```python
from build123d import *

# Parameters (mm, degrees)
F1_DEPTH = 15.875


with BuildPart() as f1:
    # F0 (on Front) → F1 (new body, symmetric)
    with BuildSketch(Plane.XZ):
        with BuildLine():
            Line((-43.1179597079, -20.6795539033), (-35.6798299226, -32.0231574202))
            ThreePointArc((-35.6798299226, -32.0231574202), (-28.999387078, -31.3506516016), (-25.4497350562, -37.0498226993))
            ThreePointArc((-25.4497350562, -37.0498226993), (-25.6219242672, -38.5185479478), (-26.1291535934, -39.9076200809))
            Line((-26.1291535934, -39.9076200809), (-15.6603085893, -45.1835936364))
            ThreePointArc((-15.6603085893, -45.1835936364), (-8.6969613087, -41.8243775437), (-3.6499608348, -47.681025418))
            Line((-3.6499608348, -47.681025418), (9.0295717487, -46.960294218))
            ThreePointArc((9.0295717487, -46.960294218), (13.3803993428, -40.5694541047), (20.6795539033, -43.1179597079))
            Line((20.6795539033, -43.1179597079), (31.2999856287, -36.1540218876))
            ThreePointArc((31.2999856287, -36.1540218876), (31.872492796, -28.4439782009), (39.4679988731, -27.0014715148))
            Line((39.4679988731, -27.0014715148), (45.1835936364, -15.6603085893))
            ThreePointArc((45.1835936364, -15.6603085893), (41.8243775437, -8.6969613087), (47.681025418, -3.6499608348))
            Line((47.681025418, -3.6499608348), (46.960294218, 9.0295717487))
            ThreePointArc((46.960294218, 9.0295717487), (40.5694541047, 13.3803993428), (43.1179597079, 20.6795539033))
            Line((43.1179597079, 20.6795539033), (36.1540218876, 31.2999856287))
            ThreePointArc((36.1540218876, 31.2999856287), (28.4439782009, 31.872492796), (27.0014715148, 39.4679988731))
            Line((27.0014715148, 39.4679988731), (15.6603085893, 45.1835936364))
            ThreePointArc((15.6603085893, 45.1835936364), (8.6969613087, 41.8243775437), (3.6499608348, 47.681025418))
            Line((3.6499608348, 47.681025418), (-9.0295717487, 46.960294218))
            ThreePointArc((-9.0295717487, 46.960294218), (-9.0218969832, 46.7801840579), (-9.0193380405, 46.599928618))
            ThreePointArc((-9.0193380405, 46.599928618), (-13.5523860225, 40.5154249107), (-20.6795539033, 43.1179597079))
            Line((-20.6795539033, 43.1179597079), (-31.2999856287, 36.1540218876))
            ThreePointArc((-31.2999856287, 36.1540218876), (-30.5256977842, 34.4890049955), (-30.2602014915, 32.6720529775))
            ThreePointArc((-30.2602014915, 32.6720529775), (-33.2803751727, 27.2651354928), (-39.4679988731, 27.0014715148))
            Line((-39.4679988731, 27.0014715148), (-45.1835936364, 15.6603085893))
            ThreePointArc((-45.1835936364, 15.6603085893), (-42.6344735333, 13.3195534454), (-41.691391018, 9.9897271266))
            ThreePointArc((-41.691391018, 9.9897271266), (-43.4256125593, 5.6288683556), (-47.681025418, 3.6499608348))
            Line((-47.681025418, 3.6499608348), (-46.960294218, -9.0295717487))
            ThreePointArc((-46.960294218, -9.0295717487), (-42.2390698471, -10.7535595818), (-40.249928618, -15.3693380405))
            ThreePointArc((-40.249928618, -15.3693380405), (-41.0127556934, -18.3869527791), (-43.1179597079, -20.6795539033))
        make_face()
        with BuildLine():
            ThreePointArc((-40.5228638212, 27.6706958124), (-43.8188886794, 22.0833623778), (-46.3490638812, 16.1100644426))
            ThreePointArc((-46.3490638812, 16.1100644426), (-45.7552417742, 15.9139166606), (-45.1835936364, 15.6603085893))
            Line((-45.1835936364, 15.6603085893), (-39.4679988731, 27.0014715148))
            ThreePointArc((-39.4679988731, 27.0014715148), (-40.0119284743, 27.3100800632), (-40.5228638212, 27.6706958124))
        make_face()
        with BuildLine():
            ThreePointArc((-21.2584815971, 44.2249574245), (-26.9065895731, 41.0341971599), (-32.0844345415, 37.1262570045))
            ThreePointArc((-32.0844345415, 37.1262570045), (-31.6682434024, 36.6594769889), (-31.2999856287, 36.1540218876))
            Line((-31.2999856287, 36.1540218876), (-20.6795539033, 43.1179597079))
            ThreePointArc((-20.6795539033, 43.1179597079), (-20.9963064816, 43.6571873513), (-21.2584815971, 44.2249574245))
        make_face()
        with BuildLine():
            ThreePointArc((3.7020936033, 48.9291774094), (-2.7846915195, 48.9899519509), (-9.2228068767, 48.1944989841))
            ThreePointArc((-9.2228068767, 48.1944989841), (-9.0957647853, 47.582160063), (-9.0295717487, 46.960294218))
            Line((-9.0295717487, 46.960294218), (3.6499608348, 47.681025418))
            ThreePointArc((3.6499608348, 47.681025418), (3.6452588769, 48.3063865448), (3.7020936033, 48.9291774094))
        make_face()
        with BuildLine():
            ThreePointArc((16.1100644426, 46.3490638812), (15.9139166606, 45.7552417742), (15.6603085893, 45.1835936364))
            Line((15.6603085893, 45.1835936364), (27.0014715148, 39.4679988731))
            ThreePointArc((27.0014715148, 39.4679988731), (27.3100800632, 40.0119284743), (27.6706958124, 40.5228638212))
            ThreePointArc((27.6706958124, 40.5228638212), (22.0833623778, 43.8188886794), (16.1100644426, 46.3490638812))
        make_face()
        with BuildLine():
            Line((36.1540218876, 31.2999856287), (43.1179597079, 20.6795539033))
            ThreePointArc((43.1179597079, 20.6795539033), (43.6571873513, 20.9963064816), (44.2249574245, 21.2584815971))
            ThreePointArc((44.2249574245, 21.2584815971), (41.0341971599, 26.9065895731), (37.1262570045, 32.0844345415))
            ThreePointArc((37.1262570045, 32.0844345415), (36.6594769889, 31.6682434024), (36.1540218876, 31.2999856287))
        make_face()
        with BuildLine():
            Line((46.960294218, 9.0295717487), (47.681025418, -3.6499608348))
            ThreePointArc((47.681025418, -3.6499608348), (48.3063865448, -3.6452588769), (48.9291774094, -3.7020936033))
            ThreePointArc((48.9291774094, -3.7020936033), (49.0340558686, -1.8523671577), (49.0690319755, 0))
            ThreePointArc((49.0690319755, 0), (48.8499094713, 4.6320884771), (48.1944989841, 9.2228068767))
            ThreePointArc((48.1944989841, 9.2228068767), (47.582160063, 9.0957647853), (46.960294218, 9.0295717487))
        make_face()
        with BuildLine():
            Line((45.1835936364, -15.6603085893), (39.4679988731, -27.0014715148))
            ThreePointArc((39.4679988731, -27.0014715148), (40.0119284743, -27.3100800632), (40.5228638212, -27.6706958124))
            ThreePointArc((40.5228638212, -27.6706958124), (43.8188886794, -22.0833623778), (46.3490638812, -16.1100644426))
            ThreePointArc((46.3490638812, -16.1100644426), (45.7552417742, -15.9139166606), (45.1835936364, -15.6603085893))
        make_face()
        with BuildLine():
            Line((31.2999856287, -36.1540218876), (20.6795539033, -43.1179597079))
            ThreePointArc((20.6795539033, -43.1179597079), (20.9963064816, -43.6571873513), (21.2584815971, -44.2249574245))
            ThreePointArc((21.2584815971, -44.2249574245), (26.9065895731, -41.0341971599), (32.0844345415, -37.1262570045))
            ThreePointArc((32.0844345415, -37.1262570045), (31.6682434024, -36.6594769889), (31.2999856287, -36.1540218876))
        make_face()
        with BuildLine():
            Line((9.0295717487, -46.960294218), (-3.6499608348, -47.681025418))
            ThreePointArc((-3.6499608348, -47.681025418), (-3.6422860692, -47.8611355781), (-3.6397271266, -48.041391018))
            ThreePointArc((-3.6397271266, -48.041391018), (-3.6553379345, -48.4863781679), (-3.7020936033, -48.9291774094))
            ThreePointArc((-3.7020936033, -48.9291774094), (2.7846915195, -48.9899519509), (9.2228068767, -48.1944989841))
            ThreePointArc((9.2228068767, -48.1944989841), (9.0957647853, -47.582160063), (9.0295717487, -46.960294218))
        make_face()
        with BuildLine():
            Line((-15.6603085893, -45.1835936364), (-26.1291535934, -39.9076200809))
            ThreePointArc((-26.1291535934, -39.9076200809), (-26.47009136, -40.501981165), (-26.8730859737, -41.0561463031))
            ThreePointArc((-26.8730859737, -41.0561463031), (-21.6539037832, -44.0326963739), (-16.1100644426, -46.3490638812))
            ThreePointArc((-16.1100644426, -46.3490638812), (-15.9139166606, -45.7552417742), (-15.6603085893, -45.1835936364))
        make_face()
        with BuildLine():
            ThreePointArc((-36.5067509859, -32.7876048449), (-36.1102701648, -32.3870137736), (-35.6798299226, -32.0231574202))
            Line((-35.6798299226, -32.0231574202), (-43.1179597079, -20.6795539033))
            ThreePointArc((-43.1179597079, -20.6795539033), (-43.6571873513, -20.9963064816), (-44.2249574245, -21.2584815971))
            ThreePointArc((-44.2249574245, -21.2584815971), (-40.7753891021, -27.2972075968), (-36.5067509859, -32.7876048449))
        make_face()
        with BuildLine():
            ThreePointArc((-48.9291774094, 3.7020936033), (-48.9899519509, -2.7846915195), (-48.1944989841, -9.2228068767))
            ThreePointArc((-48.1944989841, -9.2228068767), (-47.582160063, -9.0957647853), (-46.960294218, -9.0295717487))
            Line((-46.960294218, -9.0295717487), (-47.681025418, 3.6499608348))
            ThreePointArc((-47.681025418, 3.6499608348), (-48.3063865448, 3.6452588769), (-48.9291774094, 3.7020936033))
        make_face()
    extrude(amount=F1_DEPTH, both=True)


solid = f1.part
```
The model under review builds one solid part; all positions refer to its coordinate system, in mm. Give positions to 0.01 mm unless a question says otherwise; leave off trailing zeros. Write each loop counter-clockwise with the first axis right and the second up, starting at its lowest first coordinate (ties: lowest second). Pieces come first, ordered by that corner, then holes. Notation, with made-up numbers: M 14.5,86.5 L 32.5,86.5 A18 ccw 32.5,108.5 Z; hole C 67,78.25 d6. An arc over 180 degrees is marked long. Answer in a Markdown table with one row per item.
Item 1: Add section C-C on z = 19.5. Give the boundary of the cut face in (x, y) (3 decimals).
Check sheet entries:
| item | result |
|---|---|
| outline | M -45.028,-15.875 L 41.777,-15.875 L 41.777,15.875 L -45.028,15.875 Z |
Item 2: Add section A-A on y = -9. Give the boundary of the cut face in (x, z).
Check sheet entries:
| item | result |
|---|---|
| outline | M -48.93,3.7 A49.07 ccw -48.19,-9.22 A6.35 cw -44.22,-21.26 A49.07 ccw -36.51,-32.79 A6.35 cw -26.87,-41.06 A49.07 ccw -16.11,-46.35 A6.35 cw -3.7,-48.93 A49.07 ccw 9.22,-48.19 A6.35 cw 21.26,-44.22 A49.07 ccw 32.08,-37.13 A6.35 cw 40.52,-27.67 A49.07 ccw 46.35,-16.11 A6.35 cw 48.93,-3.7 A49.07 ccw 48.19,9.22 A6.35 cw 44.22,21.26 A49.07 ccw 37.13,32.08 A6.35 cw 27.67,40.52 A49.07 ccw 16.11,46.35 A6.35 cw 3.7,48.93 A49.07 ccw -9.22,48.19 A6.35 cw -21.26,44.22 A49.07 ccw -32.08,37.13 A6.35 cw -40.52,27.67 A49.07 ccw -46.35,16.11 A6.35 cw Z |
Item 3: For line 1 along Z through (x, y) = (44, -9); line 2 along Z through (x, y) = (-3.5, 0); line 3 along Z through (x, y) = (31, -6), list the stretches that pass through material, from the lowest coordinate up.
Check sheet entries:
| item | result |
|---|---|
| line 1 | -21.72 to -14.89, -5.09 to 9.58, 21.16 to 21.72 |
| line 2 | -48.94 to 48.94 |
| line 3 | -38.04 to -35.65, -29.7 to 30.48 |
Item 4: Draft analysis for pull direction X (two halves, no side actions). For faces 1 (the face through (8.83, -0.22, 41.8)), 2 (the face through (-2.694, -0.222, 48.995)), 3 (the face through (-40.83, -0.222, -27.216)), state which applies: +X half, -X half, draft (parallel to the pull), parting line (faces both ways), or undercut.
Check sheet entries:
| item | result |
|---|---|
| face 1 | undercut |
| face 2 | parting line |
| face 3 | -X half |
Item 5: Add section B-B on x = 7.5. Give the boundary of the cut face in (y, z) (3 decimals).
Check sheet entries:
| item | result |
|---|---|
| outline | M -15.875,-48.492 L 15.875,-48.492 L 15.875,42.2 L -15.875,42.2 Z |
Item 6: For P1, Ø4, axis at x = 22.5, y = -9.5, coming from the -Z side; P2, Ø12, axis at y = -1, z = 7, coming from the +X side; P3, Ø8, axis at x = 38, y = -1, coming from the +Z side, all flat-tipped, find the tip position at first contact; note any pin that passes through.
Check sheet entries:
| item | result |
|---|---|
| P1 | z = -44.22 |
| P2 | x = 49.06 |
| P3 | z = 32.08 |
